The model under review builds one solid part; all positions refer to its coordinate system, in mm. A direction names the side the tool comes from. Round coordinates to 2 decimals unless told otherwise and drop trailing zeros. Write each loop counter-clockwise with the first axis right and the second up, starting at its lowest first coordinate (ties: lowest second). Pieces come first, ordered by that corner, then holes. Notation, with made-up numbers: (-9, 51.25) -> (31, 51.25) arc R22 cw to (31, 83.25) -> close; hole circle Ø4 at (-7, 13). An arc over 180 degrees is marked (long way). Use CSV: the item, a comma, the result in double quotes. Start each with the question number.
1) Take a section at C-C, the plane x = -8. State how many separate pieces and enclosed holes the cut face has, then the cut area to 3 significant figures.
2) For pin 1 Ø1 at (x, y) = (-9, 26.5) entering from +Z; pin 2 Ø1.5 at (y, z) = (22.5, 56) entering from +X; pin 3 Ø15 at (x, z) = (1.5, 25.5) entering from +Y; pin 4 Ø2 at (x, z) = (0, 30.5) entering from -Y, all flat-tipped, find the tip position at first contact; note any pin that passes through.
3) Take a section at B-B, the plane y = 0. Give the boundary of the cut face in (x, z), then the cut area to 3 significant figures.
4) Mouldability with a two-part tool opening along X and no side actions: class faces 4 (the face through (-33.49, -0.36, 28.74)), 5 (the face through (-16.014, -26.786, 13.73)), 6 (the face through (19.694, 26.786, 7.67)) as released by +X, released by -X, zero draft, split by the parting line, or undercut.
5) Machinability: for faces 1 (the face through (-4, -25.3, 31)), 2 (the face through (0, -27, 11)), 3 (the face through (-33.49, -0.28, -7.95)), which of the approach directions +Z, -Z, +X, -X, +Y, -Y give a long, thin tool a straight path to every point of the face, cutting with its end or side? Answer none if there is none.
6) Take a section at A-A, the plane x = -28. Give the boundary of the cut face in (y, z), then the cut area to 3 significant figures.
7) Wall thickness on probe 1 along Z at (x, y) = (-33.1, 0); probe 2 along Y at (x, z) = (0.5, 35); probe 3 along X at (y, z) = (38.5, 33): over which ranges is each line inside the solid? List them lowest first. Write a range as [from, to].
from build123d import *

# Parameters (mm, degrees)
SKETCH013_R     = 45
PAD004_DEPTH    = 3
SKETCH014_R     = 1.65
PAD005_DEPTH    = 3
FILLET001_R     = 0.5
FILLET002_R     = 2
CHAMFER001_SIZE = 0.5
CHAMFER002_SIZE = 0.5
CHAMFER003_SIZE = 0.5
SKETCH015_R     = 1.65
POCKET007_DEPTH = 35.001
CHAMFER004_SIZE = 0.5


with BuildPart() as part:
    # Sketch013 → Pad004 (new body)
    with BuildSketch(Plane.YZ.offset(-35)):
        with Locations((0, 30.3506240158)):
            Circle(SKETCH013_R)
    extrude(amount=PAD004_DEPTH)

    # Sketch014 → Pad005 (join)
    with BuildSketch(Plane.XZ.offset(-25.3)):
        with BuildLine():
            Line((-32, 61.5), (0, 61.5))
            ThreePointArc((16.2380952381, 56.90689802), (8.4375992255, 60.3296315651), (0, 61.5))
            ThreePointArc((21, 48.38854382), (19.7287156094, 53.2680441847), (16.2380952381, 56.90689802))
            Line((21, 48.38854382), (21, 12.61145618))
            ThreePointArc((16.2380952381, 4.09310198), (19.7287156094, 7.7319558153), (21, 12.61145618))
            ThreePointArc((0, -0.5), (8.4375992255, 0.6703684349), (16.2380952381, 4.09310198))
            Line((0, -0.5), (-32, -0.5))
            Line((-32, -0.5), (-32, 61.5))
        make_face()
        with Locations((0, 30.5)):
            Circle(SKETCH014_R, mode=Mode.SUBTRACT)
        with BuildLine():
            ThreePointArc((-15.1997755633, 8.7924708263), (0, 4), (15.1997755633, 8.7924708263))
            ThreePointArc((15.1997755633, 8.7924708263), (16.0592901911, 13.6670205086), (11.1847405088, 14.5265351364))
            ThreePointArc((-11.1847405088, 14.5265351364), (0, 11), (11.1847405088, 14.5265351364))
            ThreePointArc((-11.1847405088, 14.5265351364), (-16.0592901911, 13.6670205086), (-15.1997755633, 8.7924708263))
        make_face(mode=Mode.SUBTRACT)
    pad005 = extrude(amount=-PAD005_DEPTH)

    # Mirrored003: Pad005 across XZ
    add(pad005.mirror(Plane.XZ))

    # Fillet001
    fillet001_edges = [part.edges().sort_by_distance(p)[0] for p in [
        (-16, -25.3, -0.5),
        (-16, -28.3, -0.5),
        (-16, 25.3, -0.5),
        (-16, 28.3, -0.5),
    ]]
    fillet(fillet001_edges, radius=FILLET001_R)

    # Fillet002
    fillet002_edges = [part.edges().sort_by_distance(p)[0] for p in [
        (-32, -28.3, 30.5),
        (-32, 25.3, 30.5),
    ]]
    fillet(fillet002_edges, radius=FILLET002_R)

    # Chamfer001
    chamfer001_edges = [part.edges().sort_by_distance(p)[0] for p in [
        (-32, -45, 30.350624),
        (-35, -45, 30.350624),
    ]]
    chamfer(chamfer001_edges, length=CHAMFER001_SIZE)

    # Chamfer002
    chamfer002_edges = [part.edges().sort_by_distance(p)[0] for p in [
        (0, -28.3, 11),
        (0, -25.3, 11),
        (0, 28.3, 11),
        (0, 25.3, 11),
    ]]
    chamfer(chamfer002_edges, length=CHAMFER002_SIZE)

    # Chamfer003
    chamfer003_edges = [part.edges().sort_by_distance(p)[0] for p in [
        (-1.65, 25.3, 30.5),
        (-1.65, -28.3, 30.5),
        (-1.65, -25.3, 30.5),
        (-1.65, 28.3, 30.5),
    ]]
    chamfer(chamfer003_edges, length=CHAMFER003_SIZE)

    # Sketch015 → Pocket007 (cut, through all)
    with BuildSketch(Plane.YZ):
        with Locations((0, 30.3506240158)):
            Circle(SKETCH015_R)
        with BuildLine():
            ThreePointArc((-20.85, -5.762635322), (0, -11.3493759842), (20.85, -5.762635322))
            ThreePointArc((20.85, -5.762635322), (21.4722431864, -3.4403921356), (19.15, -2.8181489491))
            ThreePointArc((-19.15, -2.8181489491), (0, -7.9493759842), (19.15, -2.8181489491))
            ThreePointArc((-19.15, -2.8181489491), (-21.4722431864, -3.4403921356), (-20.85, -5.762635322))
        make_face()
    extrude(amount=-POCKET007_DEPTH, mode=Mode.SUBTRACT)

    # Chamfer004
    chamfer004_edges = [part.edges().sort_by_distance(p)[0] for p in [
        (-32, -1.65, 30.350624),
        (-32, 0, -7.949376),
        (-35, 0, -7.949376),
        (-35, -1.65, 30.350624),
    ]]
    chamfer(chamfer004_edges, length=CHAMFER004_SIZE)


solid = part.part
Values found:
1,separate pieces,"4"
1,enclosed holes,"0"
1,area,"326 mm²"
2,pin 1,"z = 61.5"
2,pin 2,"x = -32"
2,pin 3,"y = 28.3"
2,pin 4,"through"
3,outline,"(-35, -14.15) -> (-34.5, -14.65) -> (-32.5, -14.65) -> (-32, -14.15) -> (-32, -11.85) -> (-32.5, -11.35) -> (-34.5, -11.35) -> (-35, -11.85) -> close; (-35, -7.45) -> (-34.5, -7.95) -> (-32.5, -7.95) -> (-32, -7.45) -> (-32, 28.2) -> (-32.5, 28.7) -> (-34.5, 28.7) -> (-35, 28.2) -> close; (-35, 32.5) -> (-34.5, 32) -> (-32.5, 32) -> (-32, 32.5) -> (-32, 74.85) -> (-32.5, 75.35) -> (-34.5, 75.35) -> (-35, 74.85) -> close"
3,area,"248 mm²"
4,face 4,"zero draft"
4,face 5,"undercut"
4,face 6,"released by +X"
5,face 1,"+Z, -Z, +X"
5,face 2,"+Y, -Y"
5,face 3,"+X, -X"
6,outline,"(-28.3, 0) arc R0.5 ccw to (-27.8, -0.5) -> (-25.8, -0.5) arc R0.5 ccw to (-25.3, 0) -> (-25.3, 61) arc R0.5 ccw to (-25.8, 61.5) -> (-27.8, 61.5) arc R0.5 ccw to (-28.3, 61) -> close; (25.3, 0) arc R0.5 ccw to (25.8, -0.5) -> (27.8, -0.5) arc R0.5 ccw to (28.3, 0) -> (28.3, 61) arc R0.5 ccw to (27.8, 61.5) -> (25.8, 61.5) arc R0.5 ccw to (25.3, 61) -> close"
6,area,"372 mm²"
7,probe 1,"[-14.65, -11.35], [-7.95, 28.7], [32, 75.35]"
7,probe 2,"[-28.3, -25.3], [25.3, 28.3]"
7,probe 3,"[-35, -32]"
